```python
from build123d import *

# Parameters (mm, degrees)
SKETCH1_W            = 225
SKETCH1_H            = 225
BOSS_EXTRUDE1_DEPTH  = 5
SKETCH2_W            = 18
SKETCH2_H            = 18
BOSS_EXTRUDE2_DEPTH  = 2
LPATTERN1_COUNT      = 6
LPATTERN1_PITCH      = 36
LPATTERN1_COUNT_DIR2 = 6
LPATTERN1_PITCH_DIR2 = 36


with BuildPart() as part:
    # Sketch1 → Boss-Extrude1 (new body)
    with BuildSketch(Plane(origin=(0, 0, 0), x_dir=(1, 0, 0), z_dir=(0, 1, 0))):
        Rectangle(SKETCH1_W, SKETCH1_H)
    extrude(amount=BOSS_EXTRUDE1_DEPTH)

    # Sketch2 → Boss-Extrude2 (add)
    with BuildSketch(Plane(origin=(0, 5, 0), x_dir=(1, 0, 0), z_dir=(0, 1, 0))):
        with Locations((-90, 90)):
            Rectangle(SKETCH2_W, SKETCH2_H)
    boss_extrude2 = extrude(amount=BOSS_EXTRUDE2_DEPTH)

    # LPattern1: Boss-Extrude2 6 × 6
    with Locations(*[(i * LPATTERN1_PITCH, 0, j * LPATTERN1_PITCH_DIR2) for i in range(LPATTERN1_COUNT) for j in range(LPATTERN1_COUNT_DIR2) if (i, j) != (0, 0)]):
        add(boss_extrude2)


solid = part.part
```
Work out the finished part from the listing and answer in its coordinate system (mm). Round coordinates to 2 decimals unless told otherwise and drop trailing zeros. Write each loop counter-clockwise with the first axis right and the second up, starting at its lowest first coordinate (ties: lowest second). Pieces come first, ordered by that corner, then holes.
1) Consider probe 1 along Z at (x, y) = (-54.5, 6.5); probe 2 along Y at (x, z) = (61.5, 80). Determine where each line is inside the solid, lowest interval first.
2) A cutting plane is placed at C-C on x = 38. Determine the outline of the cut face in (y, z).
3) A cutting plane is placed at B-B on x = 14.5. Determine the outline of the cut face in (y, z).
4) Flat-ended cylindrical pins translate along their axes: P1, Ø0.6, axis at y = 6.5, z = -20.5, coming from the -X side; P2, Ø0.6, axis at x = 57.5, y = 6.5, coming from the -Z side; P3, Ø0.6, axis at x = 20, y = 5.5, coming from the +Z side. Find the tip coordinate at first contact, or state that the pin passes through.
5) A cutting plane is placed at A-A on z = 94. Determine the outline of the cut face in (x, y).
Entries:
1. probe 1: z = -99 to -81, -63 to -45, -27 to -9, 9 to 27, 45 to 63, 81 to 99
1. probe 2: y = 0 to 5
2. outline: (0, -112.5) - (5, -112.5) - (5, 112.5) - (0, 112.5) - close
3. outline: (0, -112.5) - (5, -112.5) - (5, -99) - (7, -99) - (7, -81) - (5, -81) - (5, -63) - (7, -63) - (7, -45) - (5, -45) - (5, -27) - (7, -27) - (7, -9) - (5, -9) - (5, 9) - (7, 9) - (7, 27) - (5, 27) - (5, 45) - (7, 45) - (7, 63) - (5, 63) - (5, 81) - (7, 81) - (7, 99) - (5, 99) - (5, 112.5) - (0, 112.5) - close
4. P1: stops at x = -99
4. P2: stops at z = -99
4. P3: stops at z = 99
5. outline: (-112.5, 0) - (112.5, 0) - (112.5, 5) - (99, 5) - (99, 7) - (81, 7) - (81, 5) - (63, 5) - (63, 7) - (45, 7) - (45, 5) - (27, 5) - (27, 7) - (9, 7) - (9, 5) - (-9, 5) - (-9, 7) - (-27, 7) - (-27, 5) - (-45, 5) - (-45, 7) - (-63, 7) - (-63, 5) - (-81, 5) - (-81, 7) - (-99, 7) - (-99, 5) - (-112.5, 5) - close
